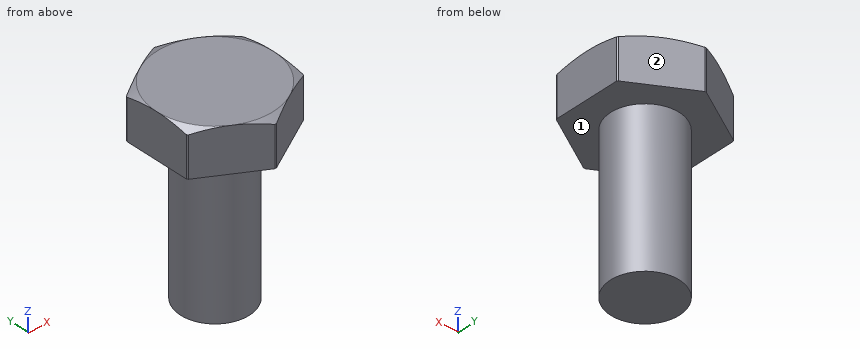
from build123d import *

# Parameters (mm, degrees)
SKETCH1_W      = 22
SKETCH1_H      = 5
EXTRUDE1_DEPTH = 6.4


with BuildPart() as part:
    # Sketch1 → Revolve1 (revolve)
    with BuildSketch(Plane(origin=(0, 0, 0), x_dir=(0, 0, -1), z_dir=(1, 0, 0))):
        with Locations((11, 2.5)):
            Rectangle(SKETCH1_W, SKETCH1_H)
    revolve(axis=Axis((0, 0, 0), (0, 0, 1)))

    # Sketch4 → Extrude1 (add)
    with BuildSketch(Plane.XY):
        Polygon((0, 9.814954576), (-8.5, 4.907477288), (-8.5, -4.907477288), (0, -9.814954576), (8.5, -4.907477288), (8.5, 4.907477288), align=None)
    extrude(amount=EXTRUDE1_DEPTH)

    # Sketch5 → Cut-Revolve3 (revolve, cut)
    with BuildSketch(Plane(origin=(0, 0, 0), x_dir=(0, 0, -1), z_dir=(1, 0, 0))):
        Polygon((-6.4, 8.5), (-5.81748528, 9.749206847), (0, 9.749206847), (0, 9.814954576), (-6.4, 9.814954576), align=None)
    revolve(axis=Axis((0, 0, 0), (0, 0, 1)), mode=Mode.SUBTRACT)


solid = part.part
The model under review builds one solid part; all positions refer to its coordinate system, in mm. Face numbers are marked on the shaded views. A direction names the side the tool comes from. Give positions to 0.01 mm unless a question says otherwise; leave off trailing zeros. Order: outer loops, then holes, each group sorted by start corner. A loop starts at its lowest first (then second) coordinate and runs counter-clockwise, first axis right, second up. Notation, with made-up numbers: M 29,-15 L 42,-15 A16 cw 42,8 Z; hole C 86,17 d10. An arc over 180 degrees is marked long. Answer in a Markdown table with one row per item. Add a question column.
1. Machinability: for the marked faces 1 and 2, which of the approach directions +Z, -Z, +X, -X, +Y, -Y give a long, thin tool a straight path to every point of the face, cutting with its end or side? Answer none if there is none.
2. Add section B-B on z = -20.5. State the section outline as (x, y) points.
3. To check wall thickness, follow line 1 along Z through (x, y) = (-4, -4); line 2 along X through (y, z) = (-6, 2.75); line 3 along X through (y, z) = (-5, 2). State the ranges of each line that lie inside material, in increasing order.
4. For pin 1 Ø1 at (x, y) = (1.5, 6) entering from -Z; pin 2 Ø5 at (x, z) = (-4, -3.5) entering from +Y; pin 3 Ø4 at (y, z) = (-7.5, 0.5) entering from +X, all flat-tipped, find the tip position at first contact; note any pin that passes through.
5. Add section A-A on z = 3. State the section outline as (x, y) points, plus the area to 3 significant figures.
The answers:
| question | item | result |
|---|---|---|
| 1 | face 1 | -Z |
| 1 | face 2 | +Z, -Z, +X, +Y |
| 2 | outline | C 0,0 d10 |
| 3 | line 1 | 0 to 6.4 |
| 3 | line 2 | -6.61 to 6.61 |
| 3 | line 3 | -8.34 to 8.34 |
| 4 | pin 1 | z = 0 |
| 4 | pin 2 | y = 4.77 |
| 4 | pin 3 | x = 7.47 |
| 5 | outline | M -8.5,-4.77 A9.75 ccw -8.38,-4.97 L -0.12,-9.75 A9.75 ccw 0.12,-9.75 L 8.38,-4.97 A9.75 ccw 8.5,-4.77 L 8.5,4.77 A9.75 ccw 8.38,4.97 L 0.12,9.75 A9.75 ccw -0.12,9.75 L -8.38,4.97 A9.75 ccw -8.5,4.77 Z |
| 5 | area | 250 mm2 |
